The listing builds one solid part. Answer for the finished solid, in the listing's coordinates (mm). Give positions to 0.01 mm unless a question says otherwise; leave off trailing zeros. Write each loop counter-clockwise with the first axis right and the second up, starting at its lowest first coordinate (ties: lowest second). Pieces come first, ordered by that corner, then holes.
Autodesk Inventor part; units mm, degrees
ref_plane "YZ Plane" through (0, 0, 0) normal (1, 0, 0) x (0, 1, 0)
ref_plane "XZ Plane" through (0, 0, 0) normal (0, 1, 0) x (-1, 0, 0)
ref_plane "XY Plane" through (0, 0, 0) normal (0, 0, 1) x (1, 0, 0)
sketch "Sketch1" plane through (0, 0, 0) normal (0, 0, 1) x (1, 0, 0)
  circle A0 centre (0, 0) radius 2.1209
  circle A1 centre (42.7862, 0) radius 2.1209
  arc A2 (0, 4.7625) -> (0, -4.7625) centre (0, 0) ccw
  arc A3 (42.7862, -4.7625) -> (42.7862, 4.7625) centre (42.7862, 0) ccw
  line L0 (0, 4.7625) -> (42.7862, 4.7625)
  line L1 (42.7862, -4.7625) -> (0, -4.7625)
  dimension "d0" = 4.2418
  dimension "d1" = 4.2418
extrude "Extrusion1" add sketch "Sketch1" along normal blind 1.5875
properties part number "joint_gusset" material "Acetal Resin, White"
Item 1: A cutting plane is placed at A-A, the plane y = 0. Give the vertices of the cut face in (x, z), plus the area to 3 significant figures.
Conclusion:
outline: (-4.76, 0) - (-2.12, 0) - (-2.12, 1.59) - (-4.76, 1.59) - close; (2.12, 0) - (40.67, 0) - (40.67, 1.59) - (2.12, 1.59) - close; (44.91, 0) - (47.55, 0) - (47.55, 1.59) - (44.91, 1.59) - close
area: 69.6 mm2
Item 2: A cutting plane is placed at C-C, the plane y = -3.5. Give the vertices of the cut face in (x, z).
Conclusion:
outline: (-3.23, 0) - (46.02, 0) - (46.02, 1.59) - (-3.23, 1.59) - close
Item 3: Determine the mould class of faces 1 (the face through (-1.683, 1.291, 0.783)), 2 (the face through (-4.76, -0.1, 0.78)), 3 (the face through (47.548, 0.105, 0.783)) for opening direction X: pulls with the +X half, pulls with the -X half, needs draft (parallel to the pull), parting line crosses it, or undercut.
Conclusion:
face 1: undercut
face 2: pulls with the -X half
face 3: pulls with the +X half
Item 4: Consider probe 1 along X at (y, z) = (-1.5, 1.4); probe 2 along X at (y, z) = (1.75, 1.55); probe 3 along Y at (x, z) = (43, 0.6). Determine where each line is inside the solid, lowest interval first.
Conclusion:
probe 1: x = -4.52 to -1.5, 1.5 to 41.29, 44.29 to 47.31
probe 2: x = -4.43 to -1.2, 1.2 to 41.59, 43.98 to 47.22
probe 3: y = -4.76 to -2.11, 2.11 to 4.76
Item 5: A cutting plane is placed at B-B, the plane z = 1.05. Give the vertices of the cut face in (x, y) (1 decimal).
Conclusion:
outline: (0, -4.8) - (42.8, -4.8) arc R4.8 ccw to (42.8, 4.8) - (0, 4.8) arc R4.8 ccw to start; hole circle Ø4.2 at (0, 0); hole circle Ø4.2 at (42.8, 0)
